Check sheet for the modelled part. Datum: model origin and axes. Units: mm. Coordinates: 2 decimals unless noted, no trailing zeros. Order: outer loops, then holes, each group sorted by start corner. A loop starts at its lowest first (then second) coordinate and runs counter-clockwise, first axis right, second up.
1. Thickness scan on line 1 (Z direction, x = -12.5, y = 3.45); line 2 (Z direction, x = 7.5, y = 1.6); line 3 (X direction, y = 0.25, z = 72.5). Record the ranges inside material, lowest first.
2. Cross-section at B-B (x = -34.5). Enter the section's corners in (y, z), then the cut area to 3 significant figures.
3. Cross-section at C-C (z = 81). Enter the section's corners in (x, y).
4. Cross-section at D-D (z = 0). Enter the section's corners in (x, y), then the cut area to 3 significant figures.
5. Cross-section at A-A (z = 29). Enter the section's corners in (x, y).
6. Gauge pin test, flat ends, axial feed: pin 1 Ø1.2 at (x, y) = (1.5, 1) entering from +Z; pin 2 Ø1.5 at (x, y) = (-18.5, 1.5) entering from -Z; pin 3 Ø2 at (y, z) = (1, 88) entering from +X. Record the tip position at first contact, or that the pin passes through.
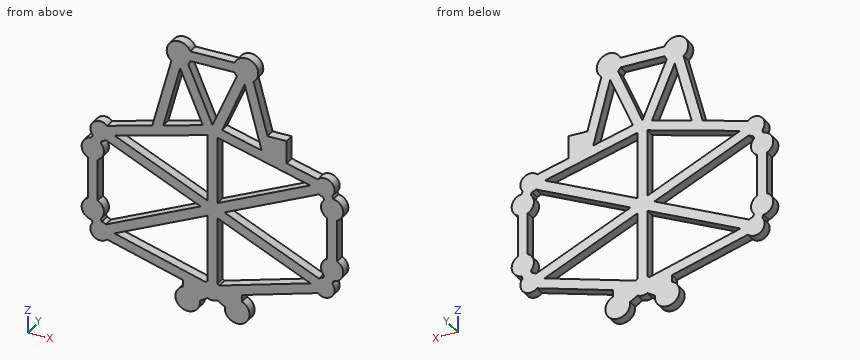
Autodesk Inventor part; units mm, degrees
ref_plane "YZ Plane" through (0, 0, 0) normal (1, 0, 0) x (0, 1, 0)
ref_plane "XZ Plane" through (0, 0, 0) normal (0, 1, 0) x (-1, 0, 0)
ref_plane "XY Plane" through (0, 0, 0) normal (0, 0, 1) x (1, 0, 0)
sketch "Sketch1" plane through (0, 0, 0) normal (0, 1, 0) x (-1, 0, 0)
  circle A0 centre (30.4866, -33.5844) radius 1.55
  circle A1 centre (30.4866, -82.5844) radius 1.55
  circle A2 centre (-31.5134, -77.3344) radius 1.55
  circle A3 centre (-31.5134, -38.8344) radius 1.55
  circle A4 centre (30.4866, -33.5844) radius 5
  circle A5 centre (30.4866, -82.5844) radius 5
  circle A6 centre (-31.5134, -77.3344) radius 5
  circle A7 centre (-31.5134, -38.8344) radius 5
  line L0 (43, 55.7856) -> (45.4, 57.1713)
  line L1 (45.4, 57.1713) -> (47.8, 55.7856)
  line L2 (47.8, 55.7856) -> (47.8, 53.0144)
  line L3 (47.8, 53.0144) -> (45.4, 51.6287)
  line L4 (45.4, 51.6287) -> (43, 53.0144)
  line L5 (43, 53.0144) -> (43, 55.7856)
  line L6 (47.8, 14.3856) -> (47.8, 11.6144)
  line L7 (47.8, 11.6144) -> (45.4, 10.2287)
  line L8 (45.4, 10.2287) -> (43, 11.6144)
  line L9 (43, 11.6144) -> (43, 14.3856)
  line L10 (43, 14.3856) -> (45.4, 15.7713)
  line L11 (45.4, 15.7713) -> (47.8, 14.3856)
  line L12 (-43, 55.7856) -> (-43, 53.0144)
  line L13 (-43, 53.0144) -> (-45.4, 51.6287)
  line L14 (-45.4, 51.6287) -> (-47.8, 53.0144)
  line L15 (-47.8, 53.0144) -> (-47.8, 55.7856)
  line L16 (-47.8, 55.7856) -> (-45.4, 57.1713)
  line L17 (-45.4, 57.1713) -> (-43, 55.7856)
  line L18 (-1.3856, 2.4) -> (1.3856, 2.4)
  line L19 (1.3856, 2.4) -> (2.7713, 0)
  line L20 (2.7713, 0) -> (1.3856, -2.4)
  line L21 (1.3856, -2.4) -> (-1.3856, -2.4)
  line L22 (-1.3856, -2.4) -> (-2.7713, 0)
  line L23 (-2.7713, 0) -> (-1.3856, 2.4)
  line L24 (-45.4, 15.7713) -> (-43, 14.3856)
  line L25 (-43, 14.3856) -> (-43, 11.6144)
  line L26 (-43, 11.6144) -> (-45.4, 10.2287)
  line L27 (-45.4, 10.2287) -> (-47.8, 11.6144)
  line L28 (-47.8, 11.6144) -> (-47.8, 14.3856)
  line L29 (-47.8, 14.3856) -> (-45.4, 15.7713)
  circle A8 centre (45.4, 54.4) radius 4
  circle A9 centre (-45.4, 54.4) radius 4
  circle A10 centre (45.4, 13) radius 4
  circle A11 centre (-45.4, 13) radius 4
  circle A12 centre (0, 0) radius 4
  line L30 (43.0778, 16.2569) -> (4.8209, 33.7)
  line L31 (4.8209, 33.7) -> (43.0778, 51.1431)
  line L32 (41.4183, 54.7827) -> (2, 36.81)
  line L33 (2, 36.81) -> (2, 63.9359)
  line L34 (41.4183, 12.6173) -> (2, 30.59)
  line L35 (2, 30.59) -> (2, 3.4641)
  line L36 (-2, 3.4641) -> (-2, 30.59)
  line L37 (-2, 30.59) -> (-41.4183, 12.6173)
  line L38 (-43.0778, 16.2569) -> (-4.8209, 33.7)
  line L39 (-4.8209, 33.7) -> (-43.0778, 51.1431)
  line L40 (-41.4183, 54.7827) -> (-2, 36.81)
  line L41 (-2, 36.81) -> (-2, 63.9359)
  line L42 (42.6203, 10.1237) -> (3.8808, -0.9691)
  line L43 (-2.7797, 2.8763) -> (-41.5192, 13.9691)
  line L44 (-42.6203, 10.1237) -> (-3.8808, -0.9691)
  line L45 (41.5192, 13.9691) -> (2.7797, 2.8763)
  line L46 (46.7546, 43.35) -> (45.1091, 46.2)
  line L47 (45.1091, 46.2) -> (46.7546, 49.05)
  line L48 (46.7546, 49.05) -> (50.0454, 49.05)
  line L49 (50.0454, 49.05) -> (51.6909, 46.2)
  line L50 (51.6909, 46.2) -> (50.0454, 43.35)
  line L51 (50.0454, 43.35) -> (46.7546, 43.35)
  line L52 (46.7546, 24.05) -> (50.0454, 24.05)
  line L53 (50.0454, 24.05) -> (51.6909, 21.2)
  line L54 (51.6909, 21.2) -> (50.0454, 18.35)
  line L55 (50.0454, 18.35) -> (46.7546, 18.35)
  line L56 (46.7546, 18.35) -> (45.1091, 21.2)
  line L57 (45.1091, 21.2) -> (46.7546, 24.05)
  line L58 (-51.6909, 21.2) -> (-50.0454, 24.05)
  line L59 (-50.0454, 24.05) -> (-46.7546, 24.05)
  line L60 (-46.7546, 24.05) -> (-45.1091, 21.2)
  line L61 (-45.1091, 21.2) -> (-46.7546, 18.35)
  line L62 (-46.7546, 18.35) -> (-50.0454, 18.35)
  line L63 (-50.0454, 18.35) -> (-51.6909, 21.2)
  line L64 (-51.6909, 46.2) -> (-50.0454, 49.05)
  line L65 (-50.0454, 49.05) -> (-46.7546, 49.05)
  line L66 (-46.7546, 49.05) -> (-45.1091, 46.2)
  line L67 (-45.1091, 46.2) -> (-46.7546, 43.35)
  line L68 (-46.7546, 43.35) -> (-50.0454, 43.35)
  line L69 (-50.0454, 43.35) -> (-51.6909, 46.2)
  line L70 (41.5368, 53.3628) -> (2, 63.9359)
  line L71 (-2, 63.9359) -> (-41.5368, 53.3628)
  line L72 (-42.5702, 57.227) -> (-30, 60.5886)
  line L73 (-30, 60.5886) -> (-30, 69.8)
  line L74 (-30, 69.8) -> (-22.2827, 69.8)
  line L75 (-22.2827, 69.8) -> (-16.6198, 90.8927)
  line L76 (16.6198, 90.8927) -> (24.3501, 62.0995)
  line L77 (24.3501, 62.0995) -> (42.5702, 57.227)
  line L78 (-11.8546, 91.95) -> (-15.1454, 91.95)
  line L79 (-15.1454, 91.95) -> (-16.7909, 94.8)
  line L80 (-16.7909, 94.8) -> (-15.1454, 97.65)
  line L81 (-15.1454, 97.65) -> (-11.8546, 97.65)
  line L82 (-11.8546, 97.65) -> (-10.2091, 94.8)
  line L83 (-10.2091, 94.8) -> (-11.8546, 91.95)
  line L84 (16.7909, 94.8) -> (15.1454, 91.95)
  line L85 (15.1454, 91.95) -> (11.8546, 91.95)
  line L86 (11.8546, 91.95) -> (10.2091, 94.8)
  line L87 (10.2091, 94.8) -> (11.8546, 97.65)
  line L88 (11.8546, 97.65) -> (15.1454, 97.65)
  line L89 (15.1454, 97.65) -> (16.7909, 94.8)
  line L90 (19.8881, 63.2928) -> (12.7566, 89.8556)
  line L91 (-12.7566, 89.8556) -> (-19.8881, 63.2928)
  line L92 (-19.8881, 63.2928) -> (-3.9062, 67.5667)
  line L93 (-3.9062, 67.5667) -> (-13.5174, 89.8)
  line L94 (19.8881, 63.2928) -> (3.9062, 67.5667)
  line L95 (3.9062, 67.5667) -> (13.5174, 89.8)
  line L96 (0, 68.6113) -> (9.8458, 91.3872)
  line L97 (0, 68.6113) -> (-9.8458, 91.3872)
  circle A13 centre (48.4, 21.2) radius 4.5
  circle A14 centre (48.4, 46.2) radius 4.5
  circle A15 centre (-48.4, 46.2) radius 4.5
  circle A16 centre (-48.4, 21.2) radius 4.5
  line L98 (50.4, 25.2311) -> (50.4, 42.1689)
  line L99 (46.4, 25.2311) -> (46.4, 42.1689)
  line L100 (48.4684, 15.5661) -> (48.8932, 16.7271)
  line L101 (44.712, 16.9404) -> (45.1367, 18.1014)
  line L102 (48.8932, 50.6729) -> (48.4684, 51.8339)
  line L103 (45.1367, 49.2986) -> (44.712, 50.4596)
  line L104 (-48.8932, 50.6729) -> (-48.4684, 51.8339)
  line L105 (-46.4, 25.2311) -> (-46.4, 42.1689)
  line L106 (-50.4, 42.1689) -> (-50.4, 25.2311)
  line L107 (-45.1367, 18.1014) -> (-44.712, 16.9404)
  line L108 (-48.4684, 15.5661) -> (-48.8932, 16.7271)
  line L109 (-45.1367, 49.2986) -> (-44.712, 50.4596)
  circle A17 centre (13.5, 94.8) radius 5
  circle A18 centre (-13.5, 94.8) radius 5
  line L110 (8.9174, 92.8) -> (-8.9174, 92.8)
  line L111 (-8.9174, 96.8) -> (8.9174, 96.8)
  line L112 (8.3546, -8.85) -> (6.7091, -6)
  line L113 (6.7091, -6) -> (8.3546, -3.15)
  line L114 (8.3546, -3.15) -> (11.6454, -3.15)
  line L115 (11.6454, -3.15) -> (13.2909, -6)
  line L116 (13.2909, -6) -> (11.6454, -8.85)
  line L117 (11.6454, -8.85) -> (8.3546, -8.85)
  line L118 (-11.6454, -3.15) -> (-8.3546, -3.15)
  line L119 (-8.3546, -3.15) -> (-6.7091, -6)
  line L120 (-6.7091, -6) -> (-8.3546, -8.85)
  line L121 (-8.3546, -8.85) -> (-11.6454, -8.85)
  line L122 (-11.6454, -8.85) -> (-13.2909, -6)
  line L123 (-13.2909, -6) -> (-11.6454, -3.15)
  circle A19 centre (10, -6) radius 5
  circle A20 centre (-10, -6) radius 5
  line L124 (5.0415, -5.3573) -> (1.9415, -3.4973)
  line L125 (-5.0415, -5.3573) -> (-1.9415, -3.4973)
  line L126 (-12, -1.4174) -> (-12, 1.3557)
  line L127 (12, -1.4174) -> (12, 1.3557)
  point P0 (0, 92.8)
  point P1 (-39.6361, 13.4299)
  point P2 (-13.0573, 88.7356)
  point P3 (13.0573, 88.7356)
  point P4 (-39.4993, 53.9077)
  point P5 (39.6361, 13.4299)
  point P6 (39.4993, 53.9077)
  dimension "d37" = 8
  dimension "d1" = 3.1
  dimension "d2" = 49
  dimension "d3" = 62
  dimension "d5" = 5.25
  dimension "d6" = 5.25
  dimension "d7" = 10
  dimension "d13" = 13
  dimension "d14" = 90.8
  dimension "d15" = 45.4
  dimension "d17" = 4
  dimension "d18" = 4
  dimension "d19" = 4
  dimension "d20" = 2
  dimension "d21" = 2
  dimension "d22" = 2
  dimension "d23" = 2
  dimension "d24" = 2
  dimension "d25" = 4
  dimension "d26" = 2
  dimension "d27" = 2
  dimension "d30" = 4
  dimension "d31" = 2
  dimension "d32" = 2
  dimension "d35" = 5.7
  dimension "d36" = 25
  dimension "d38" = 4.8
  dimension "d39" = 69.8
  dimension "d40" = 15.4
  dimension "d41" = 4
  dimension "d42" = 4
  dimension "d43" = 2
  dimension "d44" = 2
  dimension "d48" = 30
  dimension "d49" = 27
  dimension "d51" = 3
  dimension "d52" = 3
  dimension "d53" = 4
  dimension "d55" = 4
  dimension "d56" = 4
  dimension "d57" = 4
  dimension "d65" = 8.2
  dimension "d66" = 9
  dimension "d67" = 4
  dimension "d68" = 2
  dimension "d69" = 4
  dimension "d70" = 2
  dimension "d71" = 2
  dimension "d72" = 4
  dimension "d73" = 2
  dimension "d74" = 2
  dimension "d75" = 4
  dimension "d76" = 2
  dimension "d77" = 2
  dimension "d78" = 4
  dimension "d79" = 2
  dimension "d80" = 4
  dimension "d81" = 2
  dimension "d82" = 10
  dimension "d83" = 4
  dimension "d84" = 2
  dimension "d85" = 27
  dimension "d86" = 2
  dimension "d87" = 2
  dimension "d88" = 2
extrude "Extrusion1" add sketch "Sketch1" along normal blind 4 contours L0 L1 L2 L3 L4 L5 | L6 L7 L8 L9 L10 L11 | L12 L13 L14 L15 L16 L17 | L18 L19 L20 L21 L22 L23 | L24 L25 L26 L27 L28 L29 | A8 | A8 L32 L70 L31 L30 A10 L45 L34 L35 A12 L36 L37 L43 A11 L38 L39 A9 L71 L40 L72 L73 L74 L75 A18 L93 L91 L97 L96 A17 L90 L95 L76 L77 | L102 A14 L103 A8 | A8 L70 L32 | A14 | A17 | L95 L90 A17 | A14 L98 A13 L99 | A17 L110 A18 L111 | A10 | A13 | A18 | L101 A13 L100 A10 | A10 L34 L45 | A10 L42 A12 L45 L34 | A18 L91 L93 | A12 | L127 A19 L124 A12 L42 | A19 | A9 | A12 L44 A11 L37 L43 | L40 L71 A9 | A9 L109 A15 L104 | L125 A20 L126 L44 A12 | L37 A11 L43 | A15 | A20 | A11 | A15 L105 A16 L106 | A16 | L108 A16 L107 A11 | L46 L47 L48 L49 L50 L51 | L52 L53 L54 L55 L56 L57 | L58 L59 L60 L61 L62 L63 | L64 L65 L66 L67 L68 L69 | L78 L79 L80 L81 L82 L83 | L84 L85 L86 L87 L88 L89 | L112 L113 L114 L115 L116 L117 | L118 L119 L120 L121 L122 L123
properties part number "v2chassis"
Data:
1. line 1: z = -10.33 to -1.67, 1.5 to 5.66, 25.8 to 30.2, 37.2 to 41.6, 61.13 to 65.27, 87.45 to 99.7
1. line 2: z = -10.33 to 4.23, 28.08 to 32.48, 34.92 to 39.32, 62.47 to 66.61, 75.88 to 85.96, 92.8 to 96.8
1. line 3: x = -21.56 to -17.42, -6.04 to -1.68, 1.68 to 6.04, 17.42 to 21.56
2. outline: (0, 7.8) - (4, 7.8) - (4, 11.96) - (0, 11.96) - close; (0, 15.77) - (4, 15.77) - (4, 20.17) - (0, 20.17) - close; (0, 47.23) - (4, 47.23) - (4, 51.63) - (0, 51.63) - close; (0, 55.24) - (4, 55.24) - (4, 59.39) - (0, 59.39) - close
2. area: 68.4 mm2
3. outline: (-19.28, 0) - (-15.13, 0) - (-15.13, 4) - (-19.28, 4) - close; (-9.71, 0) - (-5.36, 0) - (-5.36, 4) - (-9.71, 4) - close; (5.36, 0) - (9.71, 0) - (9.71, 4) - (5.36, 4) - close; (15.13, 0) - (19.28, 0) - (19.28, 4) - (15.13, 4) - close
4. outline: (-12, 0) - (12, 0) - (12, 4) - (-12, 4) - close
4. area: 96.0 mm2
5. outline: (-50.4, 0) - (-46.4, 0) - (-46.4, 4) - (-50.4, 4) - close; (-15.13, 0) - (-5.49, 0) - (-5.49, 4) - (-15.13, 4) - close; (-2, 0) - (2, 0) - (2, 4) - (-2, 4) - close; (5.49, 0) - (15.13, 0) - (15.13, 4) - (5.49, 4) - close; (46.4, 0) - (50.4, 0) - (50.4, 4) - (46.4, 4) - close
6. pin 1: stops at z = 96.8
6. pin 2: stops at z = 3
6. pin 3: stops at x = 17.66
